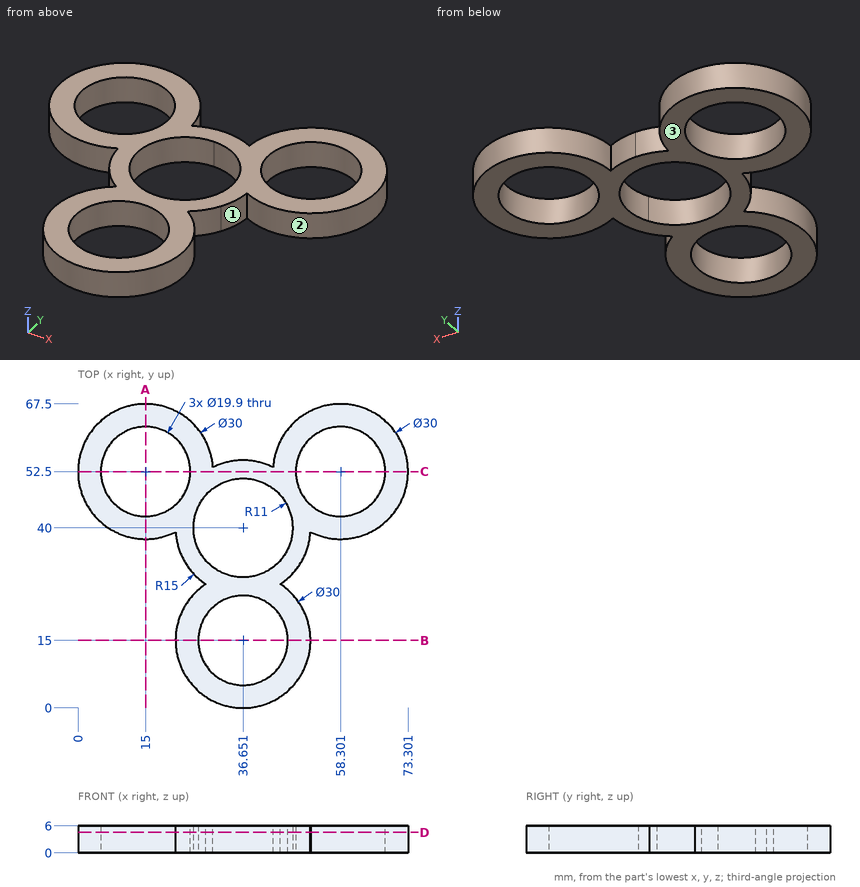
For this review, use the dimensioned drawing (mm, ordinates from the lowest corner) and the shaded views. Coordinates: 2 decimals unless noted, no trailing zeros. Loops run counter-clockwise (first coordinate to the right, second up) from the corner with the lowest first, then second, coordinate; pieces in that order, holes last.
1. Insertion check: P1, Ø1, axis at y = 17.5, z = 4.5, coming from the +X side; P2, Ø2, axis at x = 12, z = 2.5, coming from the +Y side; P3, Ø2, axis at x = 42.5, y = 20, coming from the -Z side; P4, Ø2, axis at x = 65.5, z = 2, coming from the +Y side. Each pin has a flat end and moves straight along its axis. Give the tip position at first contact, or say it passes through.
2. Add section B-B, the plane y = 15. Give the boundary of the cut face in (x, z), then the cut area to 3 significant figures.
3. Add section D-D, the plane z = 4.55. Count the separate pieces of the cut face and the enclosed holes in it, then the cut area to 3 significant figures.
4. For line 1 (Y direction, x = 15, z = 1.3); line 2 (Y direction, x = 40.5, z = 5.4) (1 decimal); line 3 (Y direction, x = 38.5, z = 3.75) (1 decimal), list the stretches that pass through material, from the lowest coordinate up.
5. Mouldability with a two-part tool opening along X and no side actions: class the marked faces 1, 2 and 3 as +X half, -X half, draft (parallel to the pull), parting line (faces both ways), or undercut.
6. Add section C-C, the plane y = 52.5. Give the boundary of the cut face in (x, z), then the cut area to 3 significant figures.
7. Add section A-A, the plane x = 15. Give the boundary of the cut face in (y, z), then the cut area to 3 significant figures.
Result:
1. P1: stops at x = 51.52
1. P2: stops at y = 67.37
1. P3: passes through
1. P4: stops at y = 66.16
2. outline: (21.65, 0) - (26.7, 0) - (26.7, 6) - (21.65, 6) - close; (46.6, 0) - (51.65, 0) - (51.65, 6) - (46.6, 6) - close
2. area: 60.6 mm2
3. separate pieces: 1
3. enclosed holes: 4
3. area: 1,350 mm2
4. line 1: y = 37.5 to 42.55, 62.45 to 67.5
4. line 2: y = 0.5 to 5.8, 24.2 to 29.7, 50.3 to 54.5
4. line 3: y = 0.1 to 5.2, 24.8 to 29.2, 50.8 to 54.9
5. face 1: undercut
5. face 2: undercut
5. face 3: draft
6. outline: (0, 0) - (5.05, 0) - (5.05, 6) - (0, 6) - close; (24.95, 0) - (48.35, 0) - (48.35, 6) - (24.95, 6) - close; (68.25, 0) - (73.3, 0) - (73.3, 6) - (68.25, 6) - close
6. area: 201 mm2
7. outline: (37.5, 0) - (42.55, 0) - (42.55, 6) - (37.5, 6) - close; (62.45, 0) - (67.5, 0) - (67.5, 6) - (62.45, 6) - close
7. area: 60.6 mm2
